Input: part model. Units: mm. Frame: model coordinates. A direction names the side the tool comes from. Give positions to 0.01 mm unless a question says otherwise; leave off trailing zeros. Loops run counter-clockwise (first coordinate to the right, second up) from the corner with the lowest first, then second, coordinate; pieces in that order, holes last. Notation, with made-up numbers: (6, 28.25) -> (48, 28.25) arc R14 cw to (48, 53.25) -> close; hole circle Ø4 at (29, 54.25). An arc over 180 degrees is marked (long way). Answer as a JSON object with one key per item and string values.
```python
from build123d import *

# Parameters (mm, degrees)
CUT_EXTRUDE1_DEPTH      = 126.928551171
CUT_EXTRUDE1_DEPTH_BACK = 126.928551171
SKETCH2_W               = 55
SKETCH2_H               = 7


with BuildPart() as part:
    # Sketch1 → Revolve1 (revolve)
    with BuildSketch(Plane(origin=(0, 0, 0), x_dir=(1, 0, 0), z_dir=(0, 1, 0)), mode=Mode.PRIVATE) as revolve1_sk:
        Polygon((120, 0), (120, 12), (100, 12), (100, 20), (30, 20), (30, 27), (0, 27), (0, 13.5), (85, 13.5), (85, 0), align=None)
    revolve(revolve1_sk.sketch.rotate(Axis((0, 0, 0), (1, 0, 0)), 180), axis=Axis((0, 0, 0), (1, 0, 0)))

    # Sketch2 → Cut-Extrude1 (cut, two sides: drawn at the far end of the back side and taken through both)
    with BuildSketch(Plane(origin=(0, 0, 0), x_dir=(1, 0, 0), z_dir=(0, 1, 0)).offset(-CUT_EXTRUDE1_DEPTH_BACK)):
        with Locations((42.5, 0)):
            Rectangle(SKETCH2_W, SKETCH2_H)
    extrude(amount=CUT_EXTRUDE1_DEPTH + CUT_EXTRUDE1_DEPTH_BACK, mode=Mode.SUBTRACT)


solid = part.part
```
Q1. Draft query along Z for faces 1 (the flat face through (85, 0, 0)), 2 (the flat face through (100, 9, -9)), 3 (the cylindrical face through (64.51, 19.524, -4.336)). Return one class per face: +Z half, -Z half, draft (parallel to the pull), parting line (faces both ways), or undercut.
Evaluation:
{"face 1": "undercut", "face 2": "draft", "face 3": "parting line"}
Q2. Ray query, line 1 along Z through (x, y) = (89.5, -16); line 2 along X through (y, z) = (0.5, -21); line 3 along Z through (x, y) = (82.5, 7) (3 decimals). Return the intervals inside material, ascending.
Evaluation:
{"line 1": "z = -12 to 12", "line 2": "x = 0 to 30", "line 3": "z = -18.735 to -11.543, 11.543 to 18.735"}
Q3. Section A-A, the plane x = 16.5. Return the cut outline in (y, z), then the cut area to 3 significant figures.
Evaluation:
{"outline": "(-26.77, -3.5) arc R27 ccw to (26.77, -3.5) -> (13.04, -3.5) arc R13.5 cw to (-13.04, -3.5) -> close; (-26.77, 3.5) -> (-13.04, 3.5) arc R13.5 cw to (13.04, 3.5) -> (26.77, 3.5) arc R27 ccw to start", "area": "1,530 mm2"}
Q4. Section B-B, the plane z = 0. Return the cut outline in (x, y).
Evaluation:
{"outline": "(0, -27) -> (15, -27) -> (15, -13.5) -> (0, -13.5) -> close; (0, 13.5) -> (15, 13.5) -> (15, 27) -> (0, 27) -> close; (70, -20) -> (100, -20) -> (100, -12) -> (120, -12) -> (120, 12) -> (100, 12) -> (100, 20) -> (70, 20) -> (70, 13.5) -> (85, 13.5) -> (85, -13.5) -> (70, -13.5) -> close"}
Q5. Access query for faces 4 (the flat face through (30, -0.4, -20.3)), 5 (the cylindrical face through (43.1, 5.17, 12.47)), 6 (the cylindrical face through (109.86, -3.604, 11.446)), 7 (the flat face through (36, 18, -3.5)). Directions: +Z, -Z, +X, -X, +Y, -Y. A direction counts if a zero-diameter tool reaches every point of the face in a straight line with its end or side. Return the directions, or none.
Evaluation:
{"face 4": "-Z, +X", "face 5": "-X", "face 6": "+X", "face 7": "+Y, -Y"}
Q6. Section D-D, the plane x = 77.5. Return the cut outline in (y, z).
Evaluation:
{"outline": "circle Ø40 at (0, 0); hole circle Ø27 at (0, 0)"}
Q7. Pin query (flat end, axial travel): pin 1 (10 mm diameter, centred on y = 8, z = -1, fed in from -X); pin 2 (2 mm diameter, centred on y = 16.5, z = 1.5, fed in from -X); pin 3 (12 mm diameter, centred on x = 97, y = -4.5, fed in from -Z); pin 4 (15 mm diameter, centred on x = 49, y = -19, fed in from +Z). Return the tip coordinate at first contact, or that it passes through.
Evaluation:
{"pin 1": "stops at x = 85", "pin 2": "stops at x = 0", "pin 3": "stops at z = -20", "pin 4": "stops at z = 16.36"}
Q8. Section C-C, the plane y = 0. Return the cut outline in (x, z).
Evaluation:
{"outline": "(0, -27) -> (30, -27) -> (30, -20) -> (100, -20) -> (100, -12) -> (120, -12) -> (120, 12) -> (100, 12) -> (100, 20) -> (30, 20) -> (30, 27) -> (0, 27) -> (0, 13.5) -> (85, 13.5) -> (85, -13.5) -> (0, -13.5) -> close"}
